Answer from the drawing. Dimensions are ordinates in mm from the lowest x, y and z of the part. Coordinates: 2 decimals unless noted, no trailing zeros. Write each loop counter-clockwise with the first axis right and the second up, starting at its lowest first coordinate (ties: lowest second). Pieces come first, ordered by that corner, then holes. Notation, with made-up numbers: (-26, -13) - (-6, -13) arc R27 ccw to (-6, 17) - close; hole circle Ø3 at (20, 3.5). An arc over 180 degrees is marked (long way). Answer as a JSON object with one key per item and string values. Group by question number.
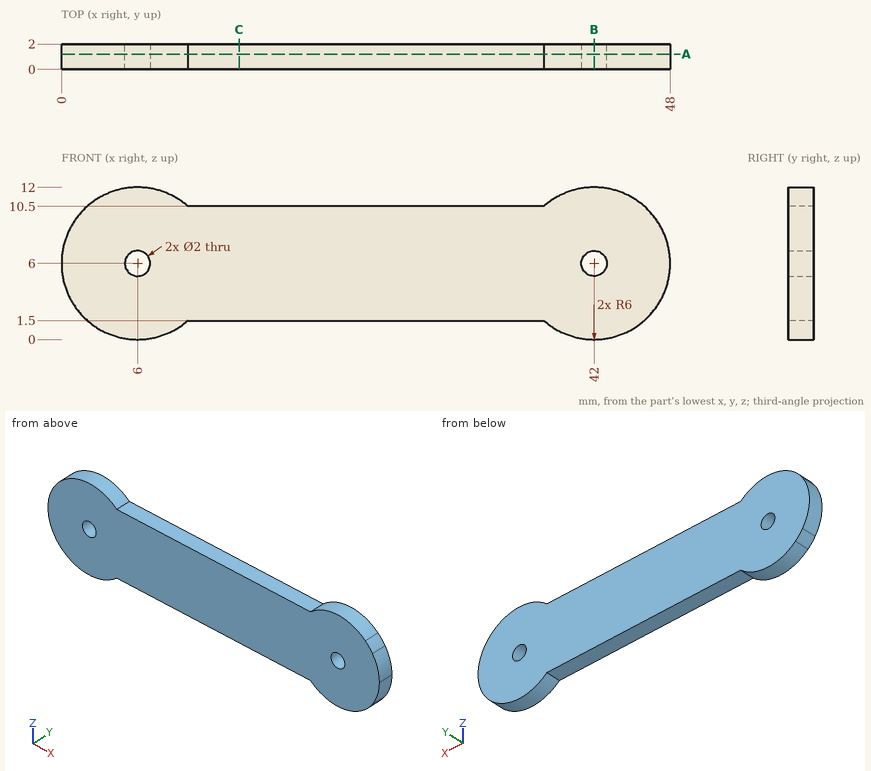
Q1. Section A-A on y = 1.2 is taken. Determine the outline of the cut face in (x, z), plus the area to 3 significant figures.
Q2. Section B-B on x = 42 is taken. Determine the outline of the cut face in (y, z).
Q3. Flat-ended cylindrical pins translate along their axes: pin 1 Ø0.6 at (x, y) = (21, 1) entering from +Z; pin 2 Ø1 at (x, y) = (29, 0.5) entering from -Z. Find the tip coordinate at first contact, or state that the pin passes through.
Q4. Consider L1, parallel to Z at x = 6, y = 0.5; L2, parallel to Z at x = 33.5, y = 1.9; L3, parallel to X at y = 0.4, z = 1.25. Determine where each line is inside the solid, lowest interval first. Write a range as from..to.
Q5. Section C-C on x = 14 is taken. Determine the outline of the cut face in (y, z).
Numbers:
{
 "1": {"outline": "(9.97, 1.5) - (38.03, 1.5) arc R6 ccw (long way) to (38.03, 10.5) - (9.97, 10.5) arc R6 ccw (long way) to start; hole circle Ø2 at (6, 6); hole circle Ø2 at (42, 6)", "area": "447 mm²"},
 "2": {"outline": "(0, 0) - (2, 0) - (2, 5) - (0, 5) - close; (0, 7) - (2, 7) - (2, 12) - (0, 12) - close"},
 "3": {"pin 1": "stops at z = 10.5", "pin 2": "stops at z = 1.5"},
 "4": {"L1": "z = 0..5, 7..12", "L2": "z = 1.5..10.5", "L3": "x = 2.33..9.67, 38.33..45.67"},
 "5": {"outline": "(0, 1.5) - (2, 1.5) - (2, 10.5) - (0, 10.5) - close"}
}
